Part model, mm, in its own coordinate system. Face numbers are marked on the shaded views. A direction names the side the tool comes from. Give positions to 0.01 mm unless a question says otherwise; leave off trailing zeros. Order: outer loops, then holes, each group sorted by start corner. A loop starts at its lowest first (then second) coordinate and runs counter-clockwise, first axis right, second up. Notation, with made-up numbers: (-25, 80) -> (-12, 80) arc R13 cw to (-12, 95) -> close; hole circle Ø9 at (43, -2.5). An arc over 180 degrees is marked (long way). Write item = value, one per line. Start each with the question number.
(1) Which spindle directions (+Z, -Z, +X, -X, +Y, -Y) get a long thin tool onto all of the face, cutting with end or side? Do the marked faces 1, 2 and 3. Say none if no direction does.
(2) Saw through at B-B, the plane x = -14.5. List the corners of the cut face in (y, z), then the cut area to 3 significant figures.
(3) Flat gauge pins, fed straight in: pin 1 (12 mm diameter, centred on y = 37.5, z = -38, fed in from -X); pin 2 (1.9 mm diameter, centred on x = -2.5, y = 9, fed in from -Z); pin 3 (5 mm diameter, centred on x = -7, y = 82.5, fed in from +Z); pin 4 (10 mm diameter, centred on y = 59, z = -14, fed in from +X). Where does each tip first touch, or does it go through?
(4) Probe line 1 along Z through (x, y) = (-16.25, 7); line 2 along Y through (x, z) = (-4, 34.5); line 3 along X through (y, z) = (41, -27). List the from-to ranges inside material, lowest first. Write a range as from..to.
(5) Saw through at A-A, the plane z = 0. List the corners of the cut face in (x, y), then the cut area to 4 significant figures.
(6) Saw through at D-D, the plane x = -2.25. List the corners of the cut face in (y, z).
(7) Saw through at C-C, the plane y = 80. List the corners of the cut face in (x, z), then the cut area to 3 significant figures.
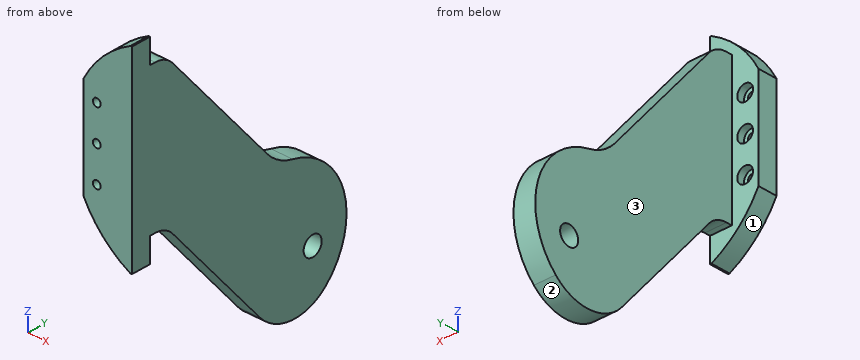
from build123d import *

# Parameters (mm, degrees)
CROQUIS1_W              = 20
CROQUIS1_H              = 80
SALIENTE_EXTRUIR2_DEPTH = 8
CORTAR_EXTRUIR1_DEPTH   = 8
CROQUIS4_R              = 4
SALIENTE_EXTRUIR3_DEPTH = 13
CROQUIS5_W              = 11
CROQUIS5_H              = 133.76595163
CORTAR_EXTRUIR2_DEPTH   = 87
CROQUIS6_R              = 1.6
CORTAR_EXTRUIR3_DEPTH   = 87
CROQUIS7_R              = 3.25
CORTAR_EXTRUIR4_DEPTH   = 3


with BuildPart() as part:
    # Croquis1 → Saliente-Extruir2 (new body)
    with BuildSketch(Plane(origin=(0, 0, 0), x_dir=(1, 0, 0), z_dir=(0, 1, 0))):
        with Locations((-10, 0)):
            Rectangle(CROQUIS1_W, CROQUIS1_H)
    extrude(amount=SALIENTE_EXTRUIR2_DEPTH)

    # Croquis2 → Cortar-Extruir1 (cut)
    with BuildSketch(Plane(origin=(0, 8, 0), x_dir=(1, 0, 0), z_dir=(0, 1, 0))):
        with BuildLine():
            ThreePointArc((-0.615528128, -40), (-11.819805153, -31.819805153), (-20, -20.615528128))
            Line((-20, -20.615528128), (-20, -40))
            Line((-20, -40), (-0.615528128, -40))
        make_face()
        with BuildLine():
            Line((-0.615528128, 40), (-20, 40))
            Line((-20, 40), (-20, 20.615528128))
            ThreePointArc((-20, 20.615528128), (-11.819805153, 31.819805153), (-0.615528128, 40))
        make_face()
    extrude(amount=-CORTAR_EXTRUIR1_DEPTH, mode=Mode.SUBTRACT)

    # Croquis4 → Saliente-Extruir3 (add)
    with BuildSketch(Plane(origin=(0, 0, 0), x_dir=(0, 0, -1), z_dir=(1, 0, 0))):
        with BuildLine():
            Line((0, 0), (30, 0))
            Line((30, 0), (30, 10.31625054))
            ThreePointArc((30, 10.31625054), (30.944105788, 14.557804503), (33.598156003, 17.998463336))
            Line((33.598156003, 17.998463336), (79.953012113, 56.627510094))
            ThreePointArc((79.953012113, 56.627510094), (87.123427128, 70.974483465), (81.447972358, 85.975807058))
            ThreePointArc((81.447972358, 85.975807058), (51.597737237, 93.799339931), (30.637508796, 71.151756681))
            ThreePointArc((30.637508796, 71.151756681), (28.203401142, 64.948074064), (23.866202653, 59.88850221))
            Line((23.866202653, 59.88850221), (-26.401843997, 17.998463336))
            ThreePointArc((-26.401843997, 17.998463336), (-29.055894212, 14.557804503), (-30, 10.31625054))
            Line((-30, 10.31625054), (-30, 0))
            Line((-30, 0), (0, 0))
        make_face()
        with Locations((65, 80)):
            Circle(CROQUIS4_R, mode=Mode.SUBTRACT)
    extrude(amount=-SALIENTE_EXTRUIR3_DEPTH)

    # Croquis5 → Cortar-Extruir2 (cut)
    with BuildSketch(Plane(origin=(0, 95, 0), x_dir=(1, 0, 0), z_dir=(0, 1, 0))):
        with Locations((-14.5, 20.266348304)):
            Rectangle(CROQUIS5_W, CROQUIS5_H)
    extrude(amount=-CORTAR_EXTRUIR2_DEPTH, mode=Mode.SUBTRACT)

    # Croquis6 → Cortar-Extruir3 (cut)
    with BuildSketch(Plane(origin=(0, 8, 0), x_dir=(1, 0, 0), z_dir=(0, 1, 0))):
        with Locations(Location((-14.5, 14.446020213, 0), (0, 0, 270))):
            Circle(CROQUIS6_R)
        with Locations(Location((-14.5, 0, 0), (0, 0, 270))):
            Circle(CROQUIS6_R)
        with Locations(Location((-14.5, -14.446020213, 0), (0, 0, 270))):
            Circle(CROQUIS6_R)
    extrude(amount=-CORTAR_EXTRUIR3_DEPTH, mode=Mode.SUBTRACT)

    # Croquis7 → Cortar-Extruir4 (cut)
    with BuildSketch(Plane(origin=(0, 8, 0), x_dir=(1, 0, 0), z_dir=(0, 1, 0))):
        with Locations(Location((-14.5, 14.446020213, 0), (0, 0, 270))):
            Circle(CROQUIS7_R)
        with Locations(Location((-14.5, 0, 0), (0, 0, 270))):
            Circle(CROQUIS7_R)
        with Locations(Location((-14.5, -14.446020213, 0), (0, 0, 270))):
            Circle(CROQUIS7_R)
    extrude(amount=-CORTAR_EXTRUIR4_DEPTH, mode=Mode.SUBTRACT)


solid = part.part
Results list:
q1.face_1 = -Z, -X, -Y
q1.face_2 = -Z, +X, -X
q1.face_3 = +Z, -Z, -X, +Y
q2.outline = (0, -28.89) -> (8, -28.89) -> (8, -17.7) -> (5, -17.7) -> (5, -16.05) -> (0, -16.05) -> close; (0, -12.85) -> (5, -12.85) -> (5, -11.2) -> (8, -11.2) -> (8, -3.25) -> (5, -3.25) -> (5, -1.6) -> (0, -1.6) -> close; (0, 1.6) -> (5, 1.6) -> (5, 3.25) -> (8, 3.25) -> (8, 11.2) -> (5, 11.2) -> (5, 12.85) -> (0, 12.85) -> close; (0, 16.05) -> (5, 16.05) -> (5, 17.7) -> (8, 17.7) -> (8, 28.89) -> (0, 28.89) -> close
q2.area = 356 mm^2
q3.pin_1 = -9
q3.pin_2 = -30
q3.pin_3 = -34.02
q3.pin_4 = through
q4.line_1 = -26.66..-17.18, -11.71..-2.74, 2.74..11.71, 17.18..26.66
q4.line_2 = 0..8
q4.line_3 = -9..0
q5.outline = (-20, 0) -> (-16.1, 0) -> (-16.1, 5) -> (-17.75, 5) -> (-17.75, 8) -> (-20, 8) -> close; (-12.9, 0) -> (0, 0) -> (0, 40) -> (-9, 40) -> (-9, 8) -> (-11.25, 8) -> (-11.25, 5) -> (-12.9, 5) -> close
q5.area = 412.5 mm^2
q6.outline = (0, -39.11) -> (8, -39.11) -> (8, -30) -> (10.32, -30) arc R10 cw to (18, -33.6) -> (56.63, -79.95) arc R20 ccw to (85.98, -81.45) arc R30 ccw to (71.15, -30.64) arc R20 cw to (59.89, -23.87) -> (18, 26.4) arc R10 ccw to (10.32, 30) -> (8, 30) -> (8, 39.11) -> (0, 39.11) -> close; hole circle Ø8 at (80, -65)
q7.outline = (-9, -85.48) -> (0, -85.48) -> (0, -69) -> (-9, -69) -> close; (-9, -61) -> (0, -61) -> (0, -34.02) -> (-9, -34.02) -> close
q7.area = 391 mm^2
